Here's how the part is built. I have some questions about the finished solid (model axes, mm). Face numbers are marked on the shaded views. A direction names the side the tool comes from. Give positions to 0.01 mm unless a question says otherwise; leave off trailing zeros. Loops run counter-clockwise (first coordinate to the right, second up) from the corner with the lowest first, then second, coordinate; pieces in that order, holes last. Notation, with made-up numbers: (25, -11.5) -> (29, -11.5) arc R13 ccw to (29, 11.5) -> close; hole circle Ø8 at (-34.75, 59.25). An arc over 180 degrees is marked (long way). Answer in a Markdown table with one row per item. Add a question column.
Item 1: If we section it at C-C (y = 8.5): Write out the boundary of the cut face in (x, z).
Item 2: If we section it at B-B (z = 4.5): Write out the boundary of the cut face in (x, y).
Item 3: For P1, Ø0.5, axis at x = -112.5, z = -0.5, coming from the +Y side; P2, Ø0.9, axis at y = 21, z = 11, coming from the -X side; P3, Ø4, axis at x = -11.5, z = 6, coming from the -Y side; P4, Ø4, axis at y = 17, z = 12.5, coming from the -X side, each with a flat end and sliding along its axis, tell me the tip position at first contact or that it passes through.
Item 4: Which directions (+Z, -Z, +X, -X, +Y, -Y) give clear straight access to the entire face, cutting with the end or side of a thin tool? Please do the marked faces 1 and 2.
Item 5: If I drill on line 1 (Z direction, x = 53, y = -13.5); line 2 (Y direction, x = 103, z = 19), over which ranges is the centre line in solid material (lowest first)?
Item 6: If we section it at A-A (x = -22.5): Write out the boundary of the cut face in (y, z), then the cut area to 3 significant figures.
```python
from build123d import *

# Parameters (mm, degrees)
SKETCH_1_W             = 240
SKETCH_1_H             = 40
SM_BASE_FLANGE_1_DEPTH = 1
SM_EDGE_FLANGE_1_DEPTH = 210


# Sheet-metal steps are written as plain solids
with BuildPart() as part:
    # Sketch 1 → 基体-法兰1 (new body)
    with BuildSketch(Plane.XY):
        Rectangle(SKETCH_1_W, SKETCH_1_H)
    extrude(amount=-SM_BASE_FLANGE_1_DEPTH)

    # 边线-法兰1 section (across the edge) → 边线-法兰1 (add)
    with BuildSketch(Plane(origin=(105, 20.7366, 0), x_dir=(0, -1, 0), z_dir=(-1, 0, 0))):
        with BuildLine():
            Line((-1, 0.7366), (-1, 29))
            Line((-1, 29), (0, 29))
            Line((0, 29), (0, 0.7366))
            ThreePointArc((0, 0.7366), (0.215745145, 0.215745145), (0.7366, 0))
            Line((0.7366, 0), (0.7366, -1))
            ThreePointArc((0.7366, -1), (-0.491361636, -0.491361636), (-1, 0.7366))
        make_face()
    extrude(amount=SM_EDGE_FLANGE_1_DEPTH)


solid = part.part
```
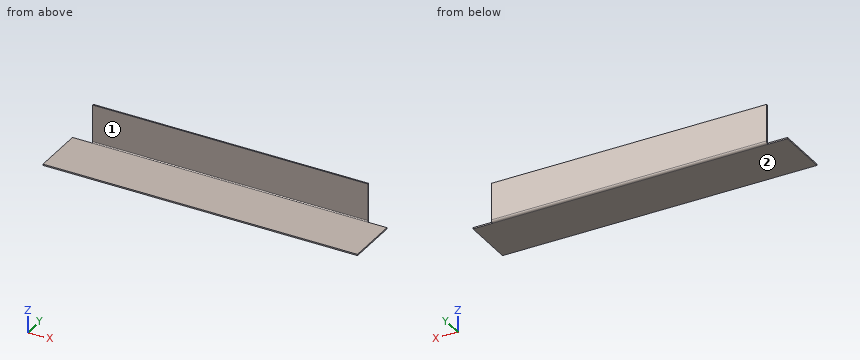
Recorded:
| question | item | result |
|---|---|---|
| 1 | outline | (-120, -1) -> (120, -1) -> (120, 0) -> (-120, 0) -> close |
| 2 | outline | (-105, 20.74) -> (105, 20.74) -> (105, 21.74) -> (-105, 21.74) -> close |
| 3 | P1 | stops at y = 20 |
| 3 | P2 | stops at x = -105 |
| 3 | P3 | stops at y = 20.74 |
| 3 | P4 | passes through |
| 4 | face 1 | +Z, +X, -X, -Y |
| 4 | face 2 | -Z, +X, -X, +Y, -Y |
| 5 | line 1 | z = -1 to 0 |
| 5 | line 2 | y = 20.74 to 21.74 |
| 6 | outline | (-20, -1) -> (20, -1) arc R1.74 ccw to (21.74, 0.74) -> (21.74, 29) -> (20.74, 29) -> (20.74, 0.74) arc R0.74 cw to (20, 0) -> (-20, 0) -> close |
| 6 | area | 70.2 mm^2 |
